Can you work these out from the model? Positions are in its coordinate system, mm. Face numbers are marked on the shaded views. A direction names the side the tool comes from. Give positions to 0.01 mm unless a question says otherwise; leave off trailing zeros. Loops run counter-clockwise (first coordinate to the right, second up) from the corner with the lowest first, then second, coordinate; pieces in that order, holes last. Notation, with made-up numbers: M -34,-13 L -8,-13 A21 ccw -8,20 Z; hole C 40,4 d8. An arc over 180 degrees is marked long. Put each result on its own line as item: value. Start each with the question number.
1) Imagine slicing it at C-C (z = 15). Write out the boundary of the cut face in (x, y), then the cut area to 3 significant figures.
2) Please list where these lines run through material, in increasing order: line 1 along Z through (x, y) = (-2.25, 44); line 2 along Z through (x, y) = (11, -1); line 3 along Z through (x, y) = (24, -2). Write a range as from..to.
3) For P1, Ø2, axis at y = 19.5, z = 14, coming from the +X side; P2, Ø3.5, axis at x = 11, z = 2.5, coming from the -Y side; P3, Ø2.5, axis at x = 14, z = -10, coming from the +Y side, each with a flat end and sliding along its axis, tell me the tip position at first contact or that it passes through.
4) For the marked faces 1 and 2, which set-ups out of +Z, -Z, +X, -X, +Y, -Y let a thin tool reach every point of the face, with its end or its side?
5) Imagine slicing it at A-A (y = 24). Write out the boundary of the cut face in (x, z).
6) Imagine slicing it at D-D (x = 27). Write out the boundary of the cut face in (y, z).
7) Imagine slicing it at B-B (x = 19). Write out the boundary of the cut face in (y, z), then the cut area to 3 significant figures.
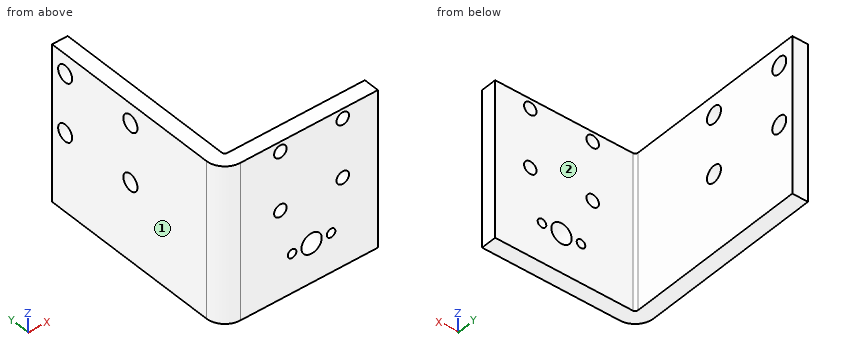
from build123d import *

# Parameters (mm, degrees)
SM_BASE_FLANGE_2_DEPTH = 20
HOLE_WIZARD_M3_1_D     = 3.2
SKETCH_24_R            = 2.6
CUT_EXTRUDE_2_DEPTH    = 67.332495807
HOLE_WIZARD_M4_1_D     = 4.3
HOLE_WIZARD_M2_1_D     = 2.2


# Sheet-metal steps are written as plain solids
with BuildPart() as part:
    # 草圖16 → 基材-凸緣2 (new, symmetric)
    with BuildSketch(Plane.XY):
        with BuildLine():
            Line((36, 0), (0.7366, 0))
            ThreePointArc((0.7366, 0), (0.215745145, 0.215745145), (0, 0.7366))
            Line((0, 0.7366), (0, 48))
            Line((0, 48), (-4, 48))
            Line((-4, 48), (-4, 0.7366))
            ThreePointArc((-4, 0.7366), (-2.61268198, -2.61268198), (0.7366, -4))
            Line((0.7366, -4), (36, -4))
            Line((36, -4), (36, 0))
        make_face()
    extrude(amount=SM_BASE_FLANGE_2_DEPTH, both=True)

    # M3 餘隙孔1 (through all)
    with Locations(Plane(origin=(0, 0, 0), x_dir=(-1, 0, 0), z_dir=(0, 1, 0))):
        with Locations((-27, 17.5), (-11, 2.5), (-11, 17.5), (-27, 2.5)):
            Hole(HOLE_WIZARD_M3_1_D / 2)

    # 草圖24 → 除料-伸長2 (cut, through all)
    with BuildSketch(Plane.XZ.offset(4)):
        with Locations(Location((19, -10, 0), (0, 0, 270))):
            Circle(SKETCH_24_R)
    extrude(amount=-CUT_EXTRUDE_2_DEPTH, mode=Mode.SUBTRACT)

    # M4 餘隙孔1 (through all)
    with Locations(Plane(origin=(0, 0, 0), x_dir=(0, 0, 1), z_dir=(1, 0, 0))):
        with Locations((0, -44), (15, -44), (15, -24), (0, -24)):
            Hole(HOLE_WIZARD_M4_1_D / 2)

    # M2 餘隙孔1 (through all)
    with Locations(Plane(origin=(0, -4, 0), x_dir=(-1, 0, 0), z_dir=(0, -1, 0))):
        with Locations((-14, 10), (-24, 10)):
            Hole(HOLE_WIZARD_M2_1_D / 2)


solid = part.part
Recorded:
1. outline: M -4,0.74 A4.74 ccw 0.74,-4 L 36,-4 L 36,0 L 0.74,0 A0.74 cw 0,0.74 L 0,21.85 L -4,21.85 Z; M -4,26.15 L 0,26.15 L 0,41.85 L -4,41.85 Z; M -4,46.15 L 0,46.15 L 0,48 L -4,48 Z
1. area: 313 mm²
2. line 1: -20..-2.15, 2.15..12.85, 17.15..20
2. line 2: -20..0.9, 4.1..15.9, 19.1..20
2. line 3: -20..-11.1, -8.9..20
3. P1: x = 0
3. P2: y = -4
3. P3: y = 0
4. face 1: +Z, -Z, -X, +Y, -Y
4. face 2: +Z, -Z, +X, +Y
5. outline: M -4,-20 L 0,-20 L 0,-2.15 L -4,-2.15 Z; M -4,2.15 L 0,2.15 L 0,12.85 L -4,12.85 Z; M -4,17.15 L 0,17.15 L 0,20 L -4,20 Z
6. outline: M -4,-20 L 0,-20 L 0,0.9 L -4,0.9 Z; M -4,4.1 L 0,4.1 L 0,15.9 L -4,15.9 Z; M -4,19.1 L 0,19.1 L 0,20 L -4,20 Z
7. outline: M -4,-20 L 0,-20 L 0,-12.6 L -4,-12.6 Z; M -4,-7.4 L 0,-7.4 L 0,20 L -4,20 Z
7. area: 139 mm²
